from build123d import *

# Parameters (mm, degrees)
BOSS_EXTRUDE1_DEPTH       = 54
CUT_EXTRUDE1_DEPTH        = 79.461774132
CUT_EXTRUDE1_DEPTH_BACK   = 79.461774132
F_3_0MM_DOWEL_HOLE1_D     = 3
F_3_0MM_DOWEL_HOLE2_D     = 2.9
F_3_0MM_DOWEL_HOLE2_DEPTH = 10
F_3_0MM_DOWEL_HOLE2_TIP   = 0.871247898
SKETCH8_W                 = 2.769274519
SKETCH8_H                 = 5
CUT_EXTRUDE2_DEPTH        = 105.672107077
SKETCH10_R                = 7.5
CUT_EXTRUDE3_DEPTH        = 10
SKETCH11_R                = 7.5
CUT_EXTRUDE4_DEPTH        = 15
CUT_EXTRUDE4_DRAFT        = -15


with BuildPart() as part:
    # Sketch1 → Boss-Extrude1 (new body)
    with BuildSketch(Plane.XY):
        Polygon((14.738209208, 40.5), (-14.738209208, 40.5), (-40, 13.43379558), (-40, 0), (-34, 0), (-34, 14), (-13, 36.5), (13, 36.5), (34, 14), (34, 0), (40, 0), (40, 13.43379558), align=None)
    extrude(amount=BOSS_EXTRUDE1_DEPTH)

    # Sketch2 → Cut-Extrude1 (cut, two sides: drawn at the far end of the back side and taken through both)
    with BuildSketch(Plane(origin=(0, 0, 0), x_dir=(0, 0, -1), z_dir=(1, 0, 0)).offset(-CUT_EXTRUDE1_DEPTH_BACK)):
        Polygon((0, 36.5), (-11, 0), (0, 0), align=None)
        Polygon((-38, 40.5), (-38, 36.5), (-54, 0), (-54, 40.5), align=None)
    extrude(amount=CUT_EXTRUDE1_DEPTH + CUT_EXTRUDE1_DEPTH_BACK, mode=Mode.SUBTRACT)

    # Ø3.0mm Dowel Hole1 (through all)
    with Locations(Plane(origin=(-8, 40.5, 4), x_dir=(0, 0, 1), z_dir=(0, 1, 0))):
        with Locations((0, 0), (0, 16), (30, 16), (30, 0)):
            Hole(F_3_0MM_DOWEL_HOLE1_D / 2)

    # Ø3.0mm Dowel Hole2
    with Locations(Plane(origin=(-37, 0, 48), x_dir=(0, 0, -1), z_dir=(0, -1, 0))):
        with Locations((0, 0), (0, 74), (31, 74), (31, 0)):
            Hole(F_3_0MM_DOWEL_HOLE2_D / 2, depth=F_3_0MM_DOWEL_HOLE2_DEPTH)
            with Locations((0, 0, -(F_3_0MM_DOWEL_HOLE2_DEPTH + F_3_0MM_DOWEL_HOLE2_TIP / 2))):  # 118° drill point
                Cone(0, F_3_0MM_DOWEL_HOLE2_D / 2, F_3_0MM_DOWEL_HOLE2_TIP, mode=Mode.SUBTRACT)

    # Sketch8 → Cut-Extrude2 (cut, through all)
    with BuildSketch(Plane.ZY.offset(40)):
        with Locations((7.807143563, 8.5)):
            Rectangle(SKETCH8_W, SKETCH8_H)
    extrude(amount=-CUT_EXTRUDE2_DEPTH, mode=Mode.SUBTRACT)

    # Sketch10 → Cut-Extrude3 (cut)
    with BuildSketch(Plane.XY.offset(38)):
        with Locations((0, 45)):
            Circle(SKETCH10_R)
    extrude(amount=-CUT_EXTRUDE3_DEPTH, mode=Mode.SUBTRACT)


with BuildPart() as cut_extrude4_tool:
    # Sketch11 → Cut-Extrude4 (with draft: the straight prism first)
    with BuildSketch(Plane.XY.offset(28)):
        with Locations((0, 45)):
            Circle(SKETCH11_R)
    extrude(amount=-CUT_EXTRUDE4_DEPTH)
    # Cut-Extrude4: the draft: its side faces are tilted about the plane it starts from
    cut_extrude4_sides = [cut_extrude4_tool.faces().sort_by_distance(p)[0] for p in [
        (-7.5, 45, 20.5),
    ]]
    draft(cut_extrude4_sides, Plane.XY.offset(28), CUT_EXTRUDE4_DRAFT)


with BuildPart() as part_1:
    add(part.part)

    # Cut-Extrude4: cut by cut_extrude4_tool
    add(cut_extrude4_tool.part, mode=Mode.SUBTRACT)


solid = part_1.part
Build history of the part. All positions in model axes, mm. A direction names the side the tool comes from. Coordinates: 2 decimals unless noted, no trailing zeros. Write each loop counter-clockwise with the first axis right and the second up, starting at its lowest first coordinate (ties: lowest second). Pieces come first, ordered by that corner, then holes. Notation, with made-up numbers: (10.5, -18) -> (29.5, -18) arc R12 cw to (29.5, 1) -> close; hole circle Ø10 at (-39, 45). An arc over 180 degrees is marked (long way). Use CSV: the item, a comma, the result in double quotes. Start each with the question number.
Q1. Cut at C-C, the plane y = 3. List the corners of the cut face in (x, z), then the cut area to 3 significant figures.
Q2. Cut at D-D, the plane y = 19. List the corners of the cut face in (x, z), then the cut area to 3 significant figures.
Q3. Cut at B-B, the plane z = 34. List the corners of the cut face in (x, y).
Q4. Pull direction X, two halves, no side cores. Call faces 1 (the flat face through (-40, 7, 30)), 2 (the flat face through (-30.56, 18.34, 45.96)), 3 (the cylindrical face through (36.12, 5.07, 46.85)): released by +X, released by -X, zero draft, split by the parting line, or undercut.
Q5. Flat gauge pins, fed straight in: pin 1 Ø3.5 at (x, z) = (8, 34) entering from -Y; pin 2 Ø2.5 at (x, z) = (8, 4) entering from +Y (1 decimal); pin 3 Ø3.5 at (x, z) = (37, 17) entering from +Y; pin 4 Ø4.5 at (x, z) = (37, 48) entering from +Y. Where does each tip first touch, or does it go through?
Q6. Drill centre lines: probe 1 along X at (y, z) = (7, 48); probe 2 along Z at (x, y) = (-37, 6); probe 3 along Z at (x, y) = (-37, 2.25). Where is each one in solid material? Low to high.
Q7. 3-axis set-ups, long thin cutter, end or side, ignore diameter. For faces 4 (the flat face through (0, 37, 38)), 5 (the cylindrical face through (-37.88, 5.07, 46.85)), 6 (the flat face through (23.35, 25.41, 23.6)), 7 (the flat face through (37, 8, 9.192)): which of +Z, -Z, +X, -X, +Y, -Y reach the whole face in a straight line?
Q8. Cut at A-A, the plane x = 8. List the corners of the cut face in (y, z), then the cut area to 3 significant figures.
Checked values:
1,outline,"(-40, 10.1) -> (-34, 10.1) -> (-34, 52.68) -> (-40, 52.68) -> close; (34, 10.1) -> (40, 10.1) -> (40, 52.68) -> (34, 52.68) -> close; hole circle Ø2.9 at (-37, 17); hole circle Ø2.9 at (-37, 48); hole circle Ø2.9 at (37, 17); hole circle Ø2.9 at (37, 48)"
1,area,"485 mm²"
2,outline,"(-34.8, 5.27) -> (-29.33, 5.27) -> (-29.33, 45.67) -> (-34.8, 45.67) -> close; (29.33, 5.27) -> (34.8, 5.27) -> (34.8, 45.67) -> (29.33, 45.67) -> close"
2,area,"442 mm²"
3,outline,"(-40, 0) -> (-34, 0) -> (-34, 14) -> (-13, 36.5) -> (-9.5, 36.5) -> (-9.5, 40.5) -> (-14.74, 40.5) -> (-40, 13.43) -> close; (-6.5, 36.5) -> (6.5, 36.5) -> (6.5, 40.5) -> (6, 40.5) arc R7.5 cw to (-6, 40.5) -> (-6.5, 40.5) -> close; (9.5, 36.5) -> (13, 36.5) -> (34, 14) -> (34, 0) -> (40, 0) -> (40, 13.43) -> (14.74, 40.5) -> (9.5, 40.5) -> close"
4,face 1,"released by -X"
4,face 2,"zero draft"
4,face 3,"undercut"
5,pin 1,"stops at y = 36.5"
5,pin 2,"passes through"
5,pin 3,"stops at y = 18.52"
5,pin 4,"stops at y = 17.97"
6,probe 1,"x = -40 to -38.45, -35.55 to -34, 34 to 35.55, 38.45 to 40"
6,probe 2,"z = 9.19 to 15.55, 18.45 to 46.55, 49.45 to 51.37"
6,probe 3,"z = 10.32 to 15.55, 18.45 to 46.55, 49.45 to 53.01"
7,face 4,"+Z, +X, -X, +Y"
7,face 5,"-Y"
7,face 6,"+Z, -Z, -Y"
7,face 7,"-Z, +X, -X, -Y"
8,outline,"(36.5, 0) -> (40.5, 0) -> (40.5, 2.5) -> (36.5, 2.5) -> close; (36.5, 5.5) -> (40.5, 5.5) -> (40.5, 32.5) -> (36.5, 32.5) -> close; (36.5, 35.5) -> (40.5, 35.5) -> (40.5, 38) -> (36.5, 38) -> close"
8,area,"128 mm²"
